Source: three-view drawing plus pictorial views. Frame: mm from the lowest corner of the part. Round coordinates to 2 decimals unless told otherwise and drop trailing zeros. Loops run counter-clockwise (first coordinate to the right, second up) from the corner with the lowest first, then second, coordinate; pieces in that order, holes last. Notation, with made-up numbers: M 26,-30 L 48,-30 A30 cw 48,-1 Z; hole C 10,76.5 d4. An arc over 180 degrees is marked long. Return JSON: item names as keys, results as strings. Group by question number.
1) Section C-C (z = 7). Count the separate pieces of the cut face and the enclosed holes in it, plus the area to 3 significant figures.
2) Section A-A (x = 70.15). Output: boundary loops of the cut face in (y, z).
3) Contact query for flat-ended pins moving along their axis: P1, Ø3.5, axis at x = 70.15, z = 6.5, coming from the -Y side; P2, Ø5, axis at x = 15.6, z = 6.5, coming from the +Y side; P3, Ø1, axis at x = 16, z = 4.5, coming from the -Y side. Output: stop coordinate, or through.
4) Material intervals for line 1 (X direction, y = 0.5, z = 5); line 2 (X direction, y = 8, z = 4.75); line 3 (X direction, y = 7.75, z = 8), sorted ascending. Write a range as from..to.
5) Section B-B (y = 9.5). Output: boundary loops of the cut face in (x, z).
6) Section D-D (z = 10.75). Output: boundary loops of the cut face in (x, y) (3 decimals).
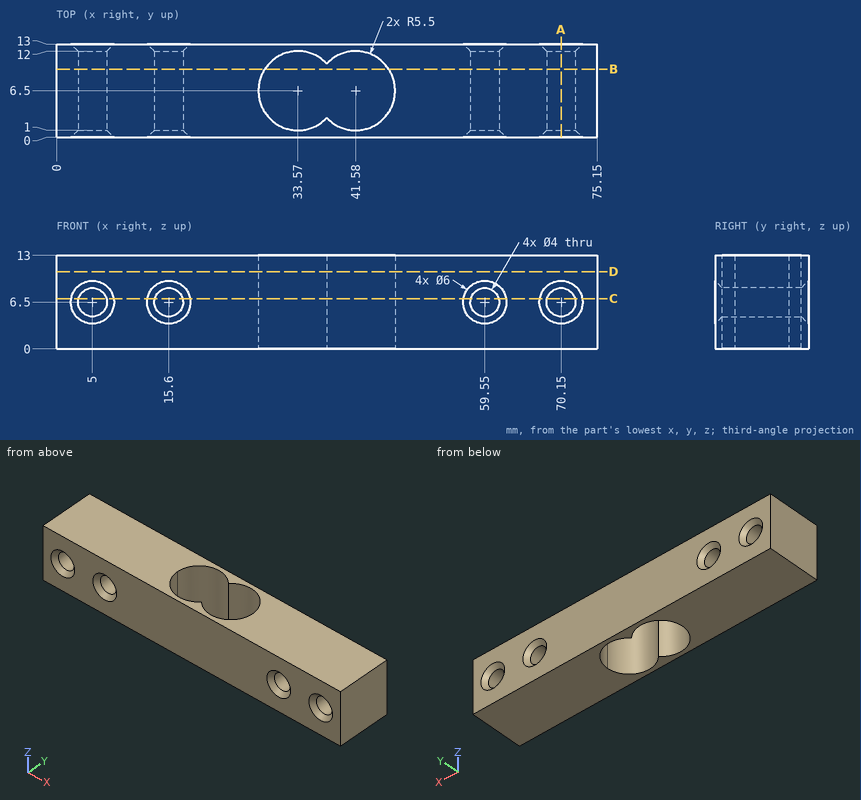
Returned:
{
 "1": {"separate pieces": "5", "enclosed holes": "1", "area": "593 mm^2"},
 "2": {"outline": "M 0,0 L 13,0 L 13,3.5 L 12,4.5 L 1,4.5 L 0,3.5 Z; M 0,9.5 L 1,8.5 L 12,8.5 L 13,9.5 L 13,13 L 0,13 Z"},
 "3": {"P1": "passes through", "P2": "stops at y = 12.5", "P3": "stops at y = 0.46"},
 "4": {"line 1": "x = 0..3, 7..13.6, 17.6..57.55, 61.55..68.15, 72.15..75.15", "line 2": "x = 0..4.03, 5.97..14.63, 16.57..28.28, 46.87..58.58, 60.52..69.18, 71.12..75.15", "line 3": "x = 0..3.68, 6.32..14.28, 16.92..28.21, 46.94..58.23, 60.87..68.83, 71.47..75.15"},
 "5": {"outline": "M 0,0 L 28.96,0 L 28.96,13 L 0,13 Z; M 46.19,0 L 75.15,0 L 75.15,13 L 46.19,13 Z; hole C 5,6.5 d4; hole C 15.6,6.5 d4; hole C 59.55,6.5 d4; hole C 70.15,6.5 d4"},
 "6": {"outline": "M 0,0 L 75.15,0 L 75.15,13 L 0,13 Z; hole M 37.575,2.73 A5.5 ccw long 37.575,10.27 A5.5 ccw long Z"}
}
